Work out the finished part from the listing and answer in its coordinate system (mm). Face numbers are marked on the shaded views. A direction names the side the tool comes from. Round coordinates to 2 decimals unless told otherwise and drop trailing zeros. Write each loop counter-clockwise with the first axis right and the second up, starting at its lowest first coordinate (ties: lowest second). Pieces come first, ordered by that corner, then holes. Notation, with made-up numbers: M -28,-26 L -5,-26 A23 cw -5,-5 Z; hole C 40,-31.5 d9. An arc over 180 degrees is marked long. Answer in a Markdown table with one row per item.
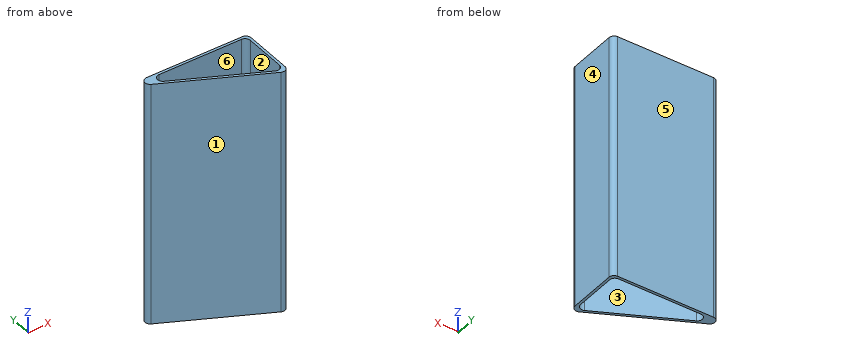
Autodesk Inventor part; units mm, degrees
ref_plane "YZ Plane" through (0, 0, 0) normal (1, 0, 0) x (0, 1, 0)
ref_plane "XZ Plane" through (0, 0, 0) normal (0, 1, 0) x (-1, 0, 0)
ref_plane "XY Plane" through (0, 0, 0) normal (0, 0, 1) x (1, 0, 0)
sketch "Sketch1" plane through (0, 0, 0) normal (0, 0, 1) x (1, 0, 0)
  line L0 (-3.175, 0) -> (-54.4382, 0)
  line L1 (-55.8581, -6.0148) -> (-4.5949, -31.6464)
  line L2 (0, -28.8066) -> (0, -3.175)
  line L3 (-1.5875, 1.5875) -> (-61.163, 1.5875)
  line L4 (-62.5829, -4.4273) -> (-3.0074, -34.215)
  line L5 (1.5875, -31.3752) -> (1.5875, -1.5875)
  arc A0 (-54.4382, 0) -> (-55.8581, -6.0148) centre (-54.4382, -3.175) ccw
  arc A1 (-61.163, 1.5875) -> (-62.5829, -4.4273) centre (-61.163, -1.5875) ccw
  arc A2 (-4.5949, -31.6464) -> (0, -28.8066) centre (-3.175, -28.8066) ccw
  arc A3 (-3.0074, -34.215) -> (1.5875, -31.3752) centre (-1.5875, -31.3752) ccw
  arc A4 (0, -3.175) -> (-3.175, 0) centre (-3.175, -3.175) ccw
  arc A5 (1.5875, -1.5875) -> (-1.5875, 1.5875) centre (-1.5875, -1.5875) ccw
  point P0 (0, 0)
  point P1 (-67.8877, 0)
  point P2 (0, -33.9439)
  point P3 (1.5875, 1.5875)
  point P4 (-74.6125, 1.5875)
  point P5 (1.5875, -36.5125)
  dimension "d0" = 1.5875
  dimension "d1" = 1.5875
  dimension "d2" = 1.5875
  dimension "d3" = 76.2
  dimension "d4" = 38.1
  dimension "d7" = 3.175
  dimension "d8" = 3.175
extrude "Extrusion1" add sketch "Sketch1" along normal blind 152.4
properties part number "BatteryMount" material "Aluminum-6061"
1. A tool of negligible diameter and unlimited length cuts with its end or side. For the marked faces 5 and 6, from which of +Z, -Z, +X, -X, +Y, -Y can it reach the whole face along a straight path? Write none if from no direction.
Calculated:
| item | result |
|---|---|
| face 5 | +Z, -Z, +X, -X, +Y |
| face 6 | +Z, -Z |
2. Consider line 1 along X through (y, z) = (-3, 118); line 2 along X through (y, z) = (-21, 136); line 3 along Y through (x, z) = (-35, 79). Determine where each line is inside the solid, lowest interval first. Write a range as from..to.
Calculated:
| item | result |
|---|---|
| line 1 | x = -64.01..-57.61, 0..1.59 |
| line 2 | x = -29.44..-25.89, 0..1.59 |
| line 3 | y = -18.22..-16.44, 0..1.59 |
3. The part is cut by section C-C (x = -23). Determine the outline of the cut face in (y, z).
Calculated:
| item | result |
|---|---|
| outline | M -24.22,0 L -22.44,0 L -22.44,152.4 L -24.22,152.4 Z; M 0,0 L 1.59,0 L 1.59,152.4 L 0,152.4 Z |
4. Given pin 1 (3 mm diameter, centred on x = -41.5, z = 85.5, fed in from -Y); pin 2 (15.5 mm diameter, centred on x = -29, z = 68, fed in from -Y); pin 3 (12 mm diameter, centred on x = -24.5, z = 50, fed in from -Y), each flat-ended and moving along its own axis, determine where each tip first touches the part or whether it passes through.
Calculated:
| item | result |
|---|---|
| pin 1 | stops at y = -15.72 |
| pin 2 | stops at y = -25.09 |
| pin 3 | stops at y = -26.47 |
5. Determine the mould class of the marked faces 1, 2, 3 and 4 for opening direction X: released by +X, released by -X, zero draft, split by the parting line, or undercut.
Calculated:
| item | result |
|---|---|
| face 1 | released by -X |
| face 2 | undercut |
| face 3 | undercut |
| face 4 | released by +X |
6. The part is cut by section A-A (y = -8.5). Determine the outline of the cut face in (x, z), plus the area to 3 significant figures.
Calculated:
| item | result |
|---|---|
| outline | M -54.44,0 L -50.89,0 L -50.89,152.4 L -54.44,152.4 Z; M 0,0 L 1.59,0 L 1.59,152.4 L 0,152.4 Z |
| area | 783 mm² |
